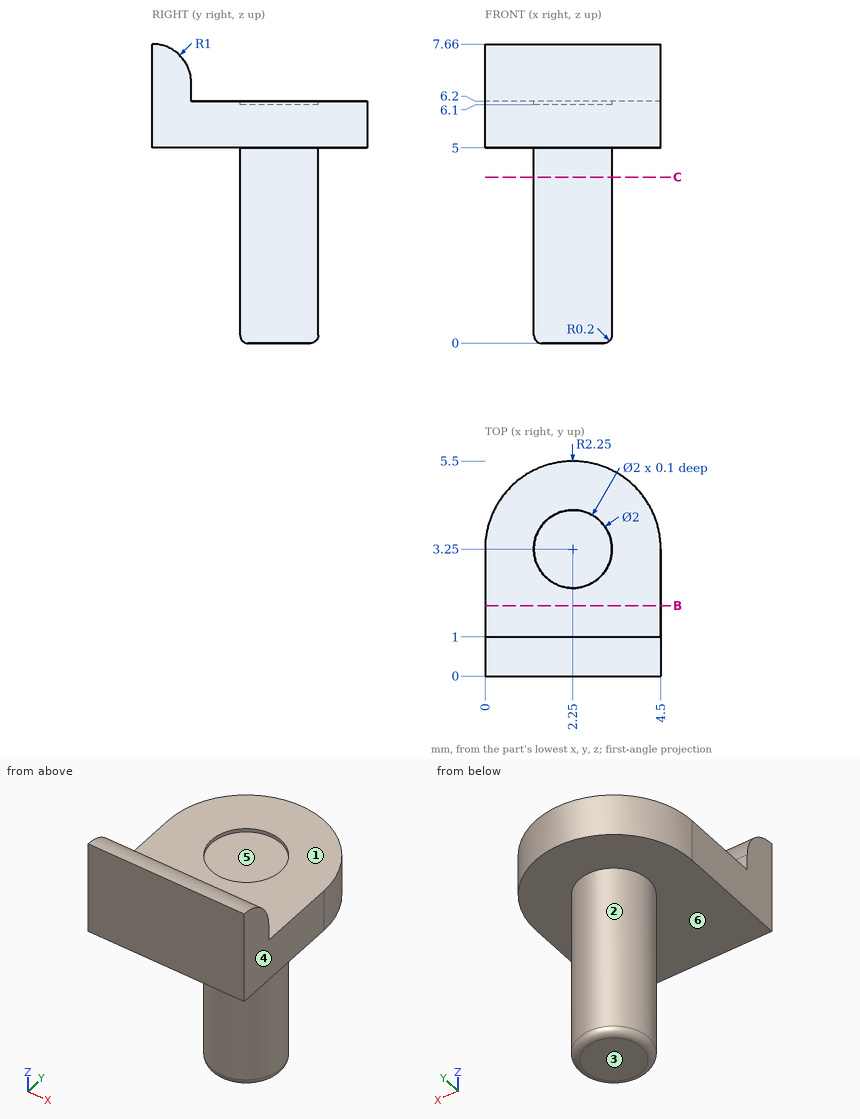
Print and shaded views of the part. All mm, measured from the part's lowest x, y and z. A direction names the side the tool comes from. Round coordinates to 2 decimals unless told otherwise and drop trailing zeros. Write each loop counter-clockwise with the first axis right and the second up, starting at its lowest first coordinate (ties: lowest second). Pieces come first, ordered by that corner, then holes. Notation, with made-up numbers: M -11,38.25 L 3,38.25 A18 ccw 3,59.25 Z; hole C 55.25,-29.5 d9. An arc over 180 degrees is marked long. Use a Markdown table: item, result. Add a question column.
1. Slice it at B-B on y = 1.8. Give the cut face in (x, z).
2. Flat gauge pins, fed straight in: P1, Ø1.5, axis at y = 0.5, z = 4, coming from the -X side (3 decimals); P2, Ø0.6, axis at x = 2, y = 3.5, coming from the +Z side; P3, Ø1, axis at x = 1.5, z = 2.5, coming from the -Y side. Where does each tip first touch, or does it go through?
3. Pull direction X, two halves, no side cores. Call the marked faces 4, 5 and 6: released by +X, released by -X, zero draft, split by the parting line, or undercut.
4. Slice it at C-C on z = 4.25. Give the cut face in (x, y), then the cut area to 3 significant figures.
5. 3-axis set-ups, long thin cutter, end or side, ignore diameter. For the marked faces 1, 2 and 3: which of +Z, -Z, +X, -X, +Y, -Y reach the whole face in a straight line?
6. Drill centre lines: probe 1 along Y at (x, z) = (2.25, 6.15); probe 2 along Z at (x, y) = (3.55, 1.55); probe 3 along X at (y, z) = (2.65, 3.25). Where is each one in solid material? Low to high.
Reply:
| question | item | result |
|---|---|---|
| 1 | outline | M 0,5 L 4.5,5 L 4.5,6.2 L 0,6.2 Z |
| 2 | P1 | passes through |
| 2 | P2 | stops at z = 6.1 |
| 2 | P3 | stops at y = 2.28 |
| 3 | face 4 | released by +X |
| 3 | face 5 | undercut |
| 3 | face 6 | zero draft |
| 4 | outline | C 2.25,3.25 d2 |
| 4 | area | 3.14 mm^2 |
| 5 | face 1 | +Z, +X, -X, +Y |
| 5 | face 2 | -Z |
| 5 | face 3 | -Z, +X, -X, +Y, -Y |
| 6 | probe 1 | y = 0 to 2.25, 4.25 to 5.5 |
| 6 | probe 2 | z = 5 to 6.2 |
| 6 | probe 3 | x = 1.45 to 3.05 |
